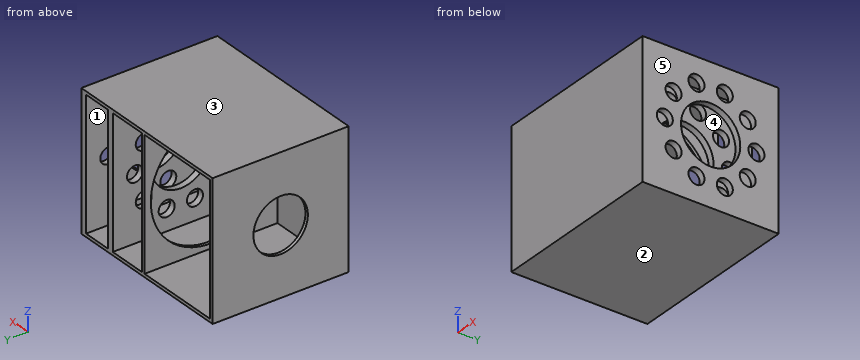
```python
from build123d import *

# Parameters (mm, degrees)
SKETCH1_W           = 110
SKETCH1_H           = 85
BOSS_EXTRUDE1_DEPTH = 85
SKETCH4_W           = 55
SKETCH4_H           = 81
SKETCH4_W_2         = 24.644091747
SKETCH4_W_3         = 18.355908253
CUT_EXTRUDE1_DEPTH  = 83
SKETCH3_R           = 18.5
CUT_EXTRUDE2_DEPTH  = 30
SKETCH2_R           = 17
CUT_EXTRUDE3_DEPTH  = 2
SKETCH6_R           = 37.5
CUT_EXTRUDE4_DEPTH  = 2
SKETCH3_3_R         = 18.5
SKETCH3_3_R_2       = 5
CUT_EXTRUDE5_DEPTH  = 40


with BuildPart() as part:
    # Sketch1 → Boss-Extrude1 (new body)
    with BuildSketch(Plane(origin=(0, 0, 0), x_dir=(1, 0, 0), z_dir=(0, 1, 0))):
        with Locations((55, 42.5)):
            Rectangle(SKETCH1_W, SKETCH1_H)
    extrude(amount=BOSS_EXTRUDE1_DEPTH)

    # Sketch4 → Cut-Extrude1 (cut)
    with BuildSketch(Plane(origin=(0, 85, 0), x_dir=(1, 0, 0), z_dir=(0, 1, 0))):
        with Locations((29.5, 42.5)):
            Rectangle(SKETCH4_W, SKETCH4_H)
        with Locations((71.322045874, 42.5)):
            Rectangle(SKETCH4_W_2, SKETCH4_H)
        with Locations((96.822045874, 42.5)):
            Rectangle(SKETCH4_W_3, SKETCH4_H)
    extrude(amount=-CUT_EXTRUDE1_DEPTH, mode=Mode.SUBTRACT)

    # Sketch3 → Cut-Extrude2 (cut)
    with BuildSketch(Plane(origin=(110, 0, 0), x_dir=(0, 0, -1), z_dir=(1, 0, 0))):
        with Locations((42.5, 42.5)):
            Circle(SKETCH3_R)
    extrude(amount=-CUT_EXTRUDE2_DEPTH, mode=Mode.SUBTRACT)

    # Sketch2 → Cut-Extrude3 (cut)
    with BuildSketch(Plane.ZY):
        with Locations((-42.5, 42.5)):
            Circle(SKETCH2_R)
    extrude(amount=-CUT_EXTRUDE3_DEPTH, mode=Mode.SUBTRACT)

    # Sketch6 → Cut-Extrude4 (cut)
    with BuildSketch(Plane.ZY.offset(-57)):
        with Locations((-42.513147441, 43.61936315)):
            Circle(SKETCH6_R)
    extrude(amount=-CUT_EXTRUDE4_DEPTH, mode=Mode.SUBTRACT)

    # Sketch3<3> → Cut-Extrude5 (cut)
    with BuildSketch(Plane(origin=(110, 0, 0), x_dir=(0, 0, -1), z_dir=(1, 0, 0))):
        with Locations((42.5, 42.5)):
            Circle(SKETCH3_3_R)
        with Locations((42.5, 71.119374851)):
            Circle(SKETCH3_3_R_2)
        with Locations((59.322046467, 65.653560623)):
            Circle(SKETCH3_3_R_2)
        with Locations((69.718642944, 51.343873197)):
            Circle(SKETCH3_3_R_2)
        with Locations((69.718642944, 33.656126803)):
            Circle(SKETCH3_3_R_2)
        with Locations((59.322046467, 19.346439377)):
            Circle(SKETCH3_3_R_2)
        with Locations((42.5, 13.880625149)):
            Circle(SKETCH3_3_R_2)
        with Locations((25.677953533, 19.346439377)):
            Circle(SKETCH3_3_R_2)
        with Locations((15.281357056, 33.656126803)):
            Circle(SKETCH3_3_R_2)
        with Locations((15.281357056, 51.343873197)):
            Circle(SKETCH3_3_R_2)
        with Locations((25.677953533, 65.653560623)):
            Circle(SKETCH3_3_R_2)
    extrude(amount=-CUT_EXTRUDE5_DEPTH, mode=Mode.SUBTRACT)


solid = part.part
```
For this review, take the finished solid that the model builds, in its own axes (mm). Face numbers are marked on the shaded views. A direction names the side the tool comes from. Coordinates: 2 decimals unless noted, no trailing zeros. Write each loop counter-clockwise with the first axis right and the second up, starting at its lowest first coordinate (ties: lowest second). Pieces come first, ordered by that corner, then holes. Notation, with made-up numbers: (1, 68.25) - (46, 68.25) arc R28 ccw to (46, 98.25) - close; hole circle Ø11 at (-6, 67.25). An arc over 180 degrees is marked (long way). Answer in a Markdown table with one row per item. Add a question column.
Q1. Tool access review of the marked faces 1 and 2: name each direction out of +Z, -Z, +X, -X, +Y, -Y from which nothing blocks a thin tool from reaching the whole face with its end or side.
Q2. For P1, Ø10, axis at y = 32.5, z = -12.5, coming from the -X side; P2, Ø9, axis at y = 51.34, z = -15.28, coming from the +X side, all flat-tipped, find the tip position at first contact; note any pin that passes through.
Q3. For probe 1 along X at (y, z) = (54.5, -25.5); probe 2 along X at (y, z) = (9.5, -22); probe 3 along Z at (x, y) = (7, 23), list the stretches that pass through material, from the lowest coordinate up.
Q4. We need section B-B, the plane z = -42.5. Count the separate pieces of the cut face and the enclosed holes in it, and give its area (3 significant figures).
Q5. We need section C-C, the plane x = 30. State the section outline as (y, z) points, and give its area (3 significant figures).
Q6. We need section A-A, the plane y = 79. State the section outline as (x, z) points.
Q7. Draft analysis for pull direction X (two halves, no side actions). For the marked faces 3, 4 and 5, state which applies: +X half, -X half, draft (parallel to the pull), parting line (faces both ways), or undercut.
Answer list:
| question | item | result |
|---|---|---|
| 1 | face 1 | +Y |
| 1 | face 2 | -Z, +X, -X, +Y, -Y |
| 2 | P1 | stops at x = 0 |
| 2 | P2 | stops at x = 2 |
| 3 | probe 1 | x = 0 to 2, 83.64 to 87.64, 106 to 110 |
| 3 | probe 2 | x = 0 to 2, 57 to 59, 83.64 to 87.64, 106 to 110 |
| 3 | probe 3 | z = -85 to -83, -2 to 0 |
| 4 | separate pieces | 9 |
| 4 | enclosed holes | 0 |
| 4 | area | 542 mm2 |
| 5 | outline | (0, -85) - (85, -85) - (85, -83) - (2, -83) - (2, -2) - (85, -2) - (85, 0) - (0, 0) - close |
| 5 | area | 502 mm2 |
| 6 | outline | (0, -85) - (110, -85) - (110, 0) - (0, 0) - close; hole (2, -83) - (57, -83) - (57, -54.94) - (59, -54.94) - (59, -83) - (83.64, -83) - (83.64, -2) - (59, -2) - (59, -30.08) - (57, -30.08) - (57, -2) - (2, -2) - close; hole (87.64, -83) - (106, -83) - (106, -2) - (87.64, -2) - close |
| 7 | face 3 | draft |
| 7 | face 4 | undercut |
| 7 | face 5 | +X half |
